Study the drawing (mm; zero at the part's minimum x, y, z) and answer. A direction names the side the tool comes from. Coordinates: 2 decimals unless noted, no trailing zeros. Loops run counter-clockwise (first coordinate to the right, second up) from the corner with the lowest first, then second, coordinate; pieces in that order, holes last. Notation, with made-up numbers: (56.25, 30.25) -> (105.25, 30.25) arc R26 cw to (105.25, 47.25) -> close; hole circle Ø7 at (80, 62). An arc over 180 degrees is marked (long way). Answer in a Markdown table with one row per item.
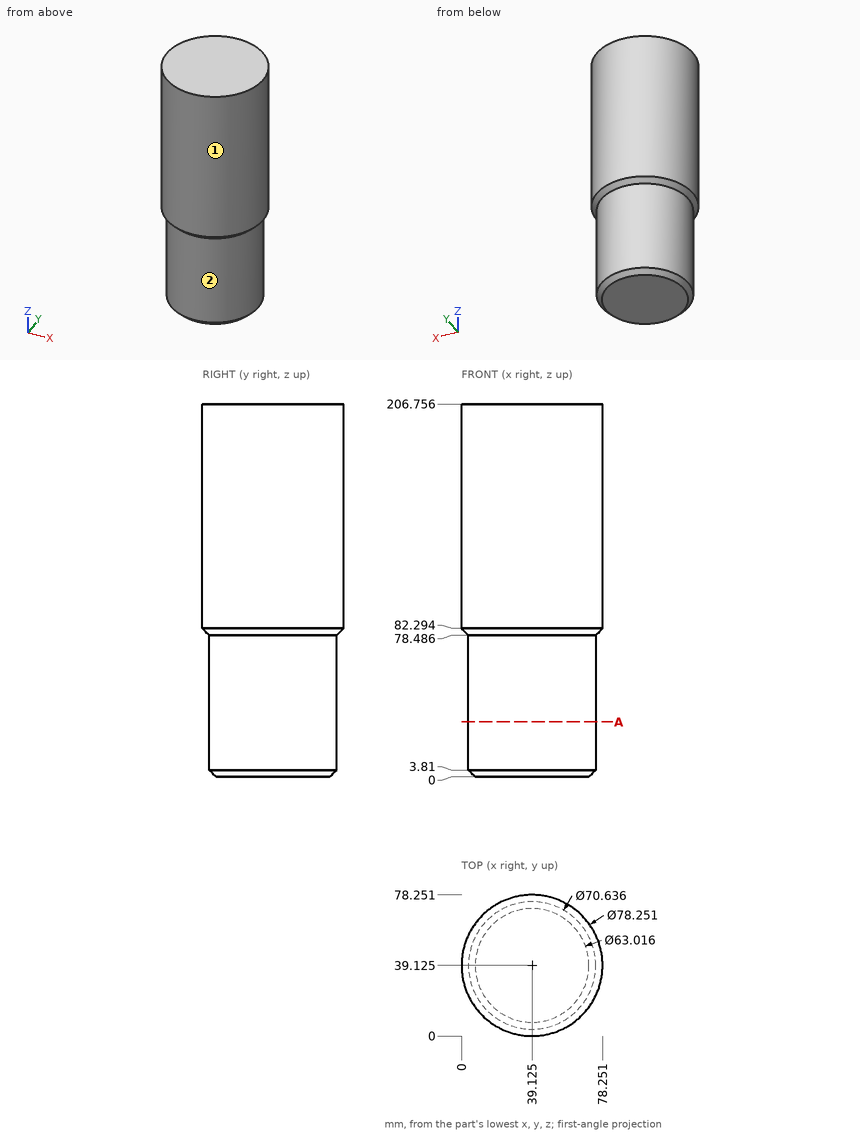
1. Find the intervals of material crossed by probe 1 along Y at (x, z) = (40.5, 33.5) (1 decimal); probe 2 along X at (y, z) = (38.5, 19.5); probe 3 along X at (y, z) = (55, 147) (1 decimal), in increasing order.
A:
| item | result |
|---|---|
| probe 1 | y = 3.8 to 74.4 |
| probe 2 | x = 3.81 to 74.44 |
| probe 3 | x = 3.4 to 74.9 |
2. A cutting plane is placed at A-A on z = 30.5. Give the vertices of the cut face in (x, y) (1 decimal), and give its area (3 significant figures).
A:
| item | result |
|---|---|
| outline | circle Ø70.6 at (39.1, 39.1) |
| area | 3,920 mm2 |
3. A tool of negligible diameter and unlimited length cuts with its end or side. For the marked faces 1 and 2, from which of +Z, -Z, +X, -X, +Y, -Y can it reach the whole face along a straight path? Write none if from no direction.
A:
| item | result |
|---|---|
| face 1 | +Z, -Z |
| face 2 | -Z |
4. Given pin 1 Ø5 at (x, z) = (70, 113) entering from -Y (1 decimal); pin 2 Ø12 at (x, z) = (11.5, 92) entering from -Y; pin 3 Ø4 at (y, z) = (56.5, 158) entering from -X, each flat-ended and moving along its own axis, determine where each tip first touches the part or whether it passes through.
A:
| item | result |
|---|---|
| pin 1 | stops at y = 12.2 |
| pin 2 | stops at y = 6.52 |
| pin 3 | stops at x = 3.15 |
